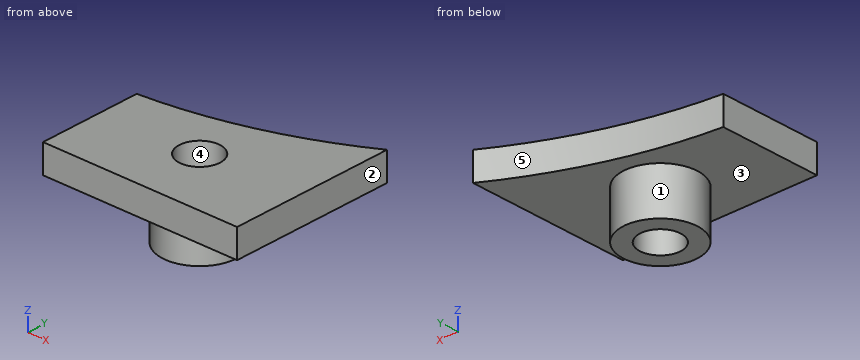
```python
from build123d import *

# Parameters (mm, degrees)
CYLINDER002_R     = 2.2
CYLINDER002_DEPTH = 20
PAD002_DEPTH      = 3
CYLINDER003_R     = 4
CYLINDER003_DEPTH = 5


with BuildPart() as hole001:
    # Cylinder002 → Cylinder002 (new body)
    with BuildSketch(Plane.XY.offset(-10)):
        Circle(CYLINDER002_R)
    extrude(amount=CYLINDER002_DEPTH)


with BuildPart() as body002:
    # Sketch003 → Pad002 (new body)
    with BuildSketch(Plane.XY):
        with BuildLine():
            Line((-10.5, -4), (-10.5, 7))
            Line((-10.5, 7), (10.5, 7))
            Line((10.5, 7), (10.5, -10.6))
            ThreePointArc((10.5, -10.6), (0.372304, -6.115398), (-10.5, -4))
        make_face()
    extrude(amount=PAD002_DEPTH)


with BuildPart() as pad_cut:
    # Cylinder003 → Cylinder003 (new body)
    with BuildSketch(Plane.XY.offset(-5)):
        Circle(CYLINDER003_R)
    extrude(amount=CYLINDER003_DEPTH)

    # Fusion001: union Body002
    add(body002.part)

    # Cut001: cut hole001
    add(hole001.part, mode=Mode.SUBTRACT)


with BuildPart() as pad_cut_mirror:
    # Part__Mirroring: instance of pad cut
    add(pad_cut.part.mirror(Plane(origin=(0, -17, 0), x_dir=(1, 0, 0), z_dir=(0, 1, 0))))


solid = pad_cut_mirror.part
```
The model under review builds one solid part; all positions refer to its coordinate system, in mm. Face numbers are marked on the shaded views. A direction names the side the tool comes from. Round coordinates to 2 decimals unless told otherwise and drop trailing zeros. Order: outer loops, then holes, each group sorted by start corner. A loop starts at its lowest first (then second) coordinate and runs counter-clockwise, first axis right, second up. Notation, with made-up numbers: (37, 41.5) - (70, 41.5) arc R4 cw to (70, 47.5) - close; hole circle Ø10 at (-36, 8). An arc over 180 degrees is marked (long way). Answer in a Markdown table with one row per item.
(1) Take a section at C-C on z = 0.25. Write out the cut boundary in (x, y).
Result set:
| item | result |
|---|---|
| outline | (-10.5, -41) - (10.5, -41) - (10.5, -23.4) arc R49.4 cw to (-10.5, -30) - close; hole circle Ø4.4 at (0, -34) |
(2) Clearance check with flat-ended pins moving along their axes: P1, Ø3, axis at x = 5, y = -39, coming from the -Z side; P2, Ø2, axis at y = -32.5, z = -4, coming from the +X side; P3, Ø1, axis at x = 6, z = 1, coming from the +Y side; P4, Ø8, axis at x = 0, y = -35, coming from the -Z side. State where each tip first meets the part, or that it passes through.
Result set:
| item | result |
|---|---|
| P1 | stops at z = 0 |
| P2 | stops at x = 3.97 |
| P3 | stops at y = -25.5 |
| P4 | stops at z = -5 |
(3) Take a section at A-A on x = 0. Write out the cut boundary in (y, z).
Result set:
| item | result |
|---|---|
| outline | (-41, 0) - (-38, 0) - (-38, -5) - (-36.2, -5) - (-36.2, 3) - (-41, 3) - close; (-31.8, -5) - (-30, -5) - (-30, 0) - (-28, 0) - (-28, 3) - (-31.8, 3) - close |
(4) Mouldability with a two-part tool opening along Y and no side actions: class the marked faces 3, 4 and 5 as released by +Y, released by -Y, zero draft, split by the parting line, or undercut.
Result set:
| item | result |
|---|---|
| face 3 | zero draft |
| face 4 | undercut |
| face 5 | released by +Y |
(5) For line 1 (Y direction, x = 0, z = -1); line 2 (Z direction, x = 7.25, y = -35); line 3 (Y direction, x = 0, z = 0.75), list the stretches that pass through material, from the lowest coordinate up. Write a range as from..to.
Result set:
| item | result |
|---|---|
| line 1 | y = -38..-36.2, -31.8..-30 |
| line 2 | z = 0..3 |
| line 3 | y = -41..-36.2, -31.8..-28 |
(6) Machinability: for the marked faces 1 and 2, which of the approach directions +Z, -Z, +X, -X, +Y, -Y give a long, thin tool a straight path to every point of the face, cutting with its end or side? Answer none if there is none.
Result set:
| item | result |
|---|---|
| face 1 | -Z |
| face 2 | +Z, -Z, +X, +Y, -Y |
(7) Take a section at D-D on x = -3.25. Write out the cut boundary in (y, z).
Result set:
| item | result |
|---|---|
| outline | (-41, 0) - (-36.33, 0) - (-36.33, -5) - (-31.67, -5) - (-31.67, 0) - (-28.87, 0) - (-28.87, 3) - (-41, 3) - close |
(8) Take a section at B-B on y = -34. Write out the cut boundary in (x, z).
Result set:
| item | result |
|---|---|
| outline | (-10.5, 0) - (-4, 0) - (-4, -5) - (-2.2, -5) - (-2.2, 3) - (-10.5, 3) - close; (2.2, -5) - (4, -5) - (4, 0) - (10.5, 0) - (10.5, 3) - (2.2, 3) - close |
